from build123d import *

# Parameters (mm, degrees)
SKETCH2_R           = 2.54
BOSS_EXTRUDE1_DEPTH = 38.1
CHAMFER1_SIZE       = 2.38
CHAMFER1_SIZE2      = 1.927285999
SKETCH3_R           = 3.81
BOSS_EXTRUDE2_DEPTH = 0.635


with BuildPart() as part:
    # Sketch2 → Boss-Extrude1 (new body)
    with BuildSketch(Plane(origin=(0, 0, 0), x_dir=(1, 0, 0), z_dir=(0, 1, 0))):
        Circle(SKETCH2_R)
    extrude(amount=BOSS_EXTRUDE1_DEPTH)

    # Chamfer1
    chamfer1_edges = [part.edges().sort_by_distance(p)[0] for p in [
        (-2.54, 38.1, 0),
    ]]
    chamfer1_side = [part.faces().sort_by_distance(p)[0] for p in [
        (-2.54, 19.05, 0),
    ]]
    chamfer(chamfer1_edges, length=CHAMFER1_SIZE, length2=CHAMFER1_SIZE2, reference=chamfer1_side[0])

    # Sketch3 → Boss-Extrude2 (add)
    with BuildSketch(Plane(origin=(0, 0, 0), x_dir=(-1, 0, 0), z_dir=(0, -1, 0))):
        Circle(SKETCH3_R)
    extrude(amount=BOSS_EXTRUDE2_DEPTH)


solid = part.part
Read the model definition and answer for the solid it produces. Units are mm, in the model's axes. A direction names the side the tool comes from. Coordinates: 2 decimals unless noted, no trailing zeros. Loops run counter-clockwise (first coordinate to the right, second up) from the corner with the lowest first, then second, coordinate; pieces in that order, holes last. Notation, with made-up numbers: (10, 7) -> (35, 7) arc R19 ccw to (35, 21) -> close; hole circle Ø3 at (77.5, 62). An arc over 180 degrees is marked (long way). Write item = value, one per line. Start each with the question number.
1) The part is cut by section D-D, the plane x = 3. Determine the outline of the cut face in (y, z) (3 decimals), plus the area to 3 significant figures.
2) For faces 1 (the face through (0, -0.635, 0)), 2 (the face through (0, 0, -3)), determine the directions among +Z, -Z, +X, -X, +Y, -Y from which every point of the face is accessible in a straight line to the end or side of a thin tool.
3) Find the intervals of material crossed by L1, parallel to Y at x = 2.25, z = -3 (3 decimals); L2, parallel to X at y = 2, z = 0, in increasing order. Write a range as from..to.
4) The part is cut by section C-C, the plane y = 5.5. Determine the outline of the cut face in (x, z).
5) Given P1, Ø2.5, axis at x = -1.5, z = -1.5, coming from the +Y side; P2, Ø4, axis at y = 14.5, z = 2, coming from the +X side; P3, Ø1, axis at x = 0.5, y = 22, coming from the -Z side, each flat-ended and moving along its own axis, determine where each tip first touches the part or whether it passes through.
6) The part is cut by section B-B, the plane z = 0. Determine the outline of the cut face in (x, y) (3 decimals), plus the area to 3 significant figures.
7) The part is cut by section A-A, the plane x = 0. Determine the outline of the cut face in (y, z) (3 decimals).
Result:
q1.outline = (-0.635, -2.349) -> (0, -2.349) -> (0, 2.349) -> (-0.635, 2.349) -> close
q1.area = 2.98 mm²
q2.face_1 = +Z, -Z, +X, -X, -Y
q2.face_2 = +Y
q3.L1 = -0.635..0
q3.L2 = -2.54..2.54
q4.outline = circle Ø5.08 at (0, 0)
q5.P1 = 37.78
q5.P2 = 2.54
q5.P3 = -2.54
q6.outline = (-3.81, -0.635) -> (3.81, -0.635) -> (3.81, 0) -> (2.54, 0) -> (2.54, 35.72) -> (0.613, 38.1) -> (-0.613, 38.1) -> (-2.54, 35.72) -> (-2.54, 0) -> (-3.81, 0) -> close
q6.area = 194 mm²
q7.outline = (-0.635, -3.81) -> (0, -3.81) -> (0, -2.54) -> (35.72, -2.54) -> (38.1, -0.613) -> (38.1, 0.613) -> (35.72, 2.54) -> (0, 2.54) -> (0, 3.81) -> (-0.635, 3.81) -> close
